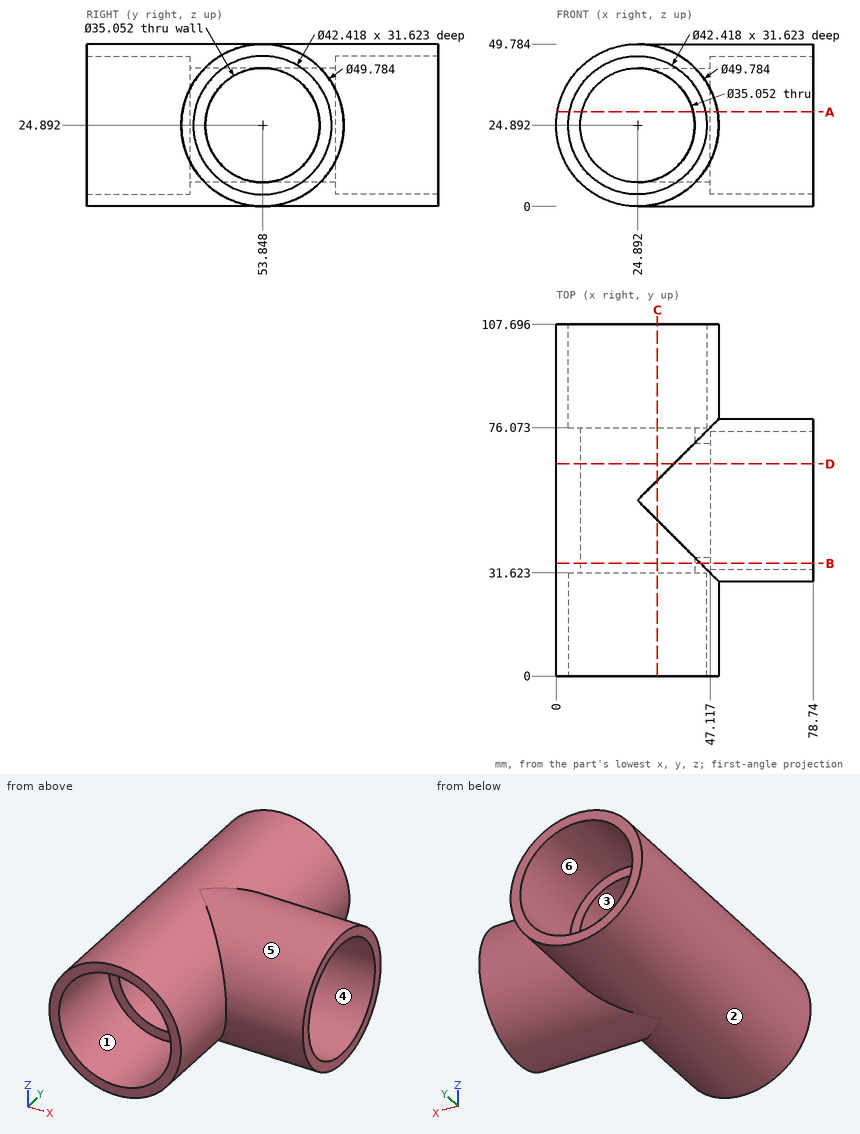
Drawing for the job (mm, zero at the part's lowest x, y, z). A direction names the side the tool comes from. Give positions to 0.01 mm unless a question says otherwise; leave off trailing zeros. Loops run counter-clockwise (first coordinate to the right, second up) from the corner with the lowest first, then second, coordinate; pieces in that order, holes last.
(1) Band-saw the part on A-A (z = 29). Write the cut outline in (x, y).
Return value:
outline: (0.34, 0) - (4.08, 0) - (4.08, 31.62) - (7.85, 31.62) - (7.85, 76.07) - (4.08, 76.07) - (4.08, 107.7) - (0.34, 107.7) - close; (41.93, 31.62) - (45.7, 31.62) - (45.7, 0) - (49.44, 0) - (49.44, 29.3) - (78.74, 29.3) - (78.74, 33.04) - (47.12, 33.04) - (47.12, 36.81) - (41.93, 36.81) - close; (41.93, 70.89) - (47.12, 70.89) - (47.12, 74.66) - (78.74, 74.66) - (78.74, 78.4) - (49.44, 78.4) - (49.44, 107.7) - (45.7, 107.7) - (45.7, 76.07) - (41.93, 76.07) - close
(2) Band-saw the part on C-C (x = 31). Write the cut outline in (y, z), and give its area (3 significant figures).
Return value:
outline: (0, 0.76) - (47.74, 0.76) arc R24.89 ccw to (59.96, 0.76) - (107.7, 0.76) - (107.7, 4.58) - (76.07, 4.58) - (76.07, 8.46) - (59.96, 8.46) arc R17.53 cw to (47.74, 8.46) - (31.62, 8.46) - (31.62, 4.58) - (0, 4.58) - close; (0, 45.2) - (31.62, 45.2) - (31.62, 41.32) - (47.74, 41.32) arc R17.53 cw to (59.96, 41.32) - (76.07, 41.32) - (76.07, 45.2) - (107.7, 45.2) - (107.7, 49.02) - (59.96, 49.02) arc R24.89 ccw to (47.74, 49.02) - (0, 49.02) - close
area: 1,160 mm2
(3) Drill centre lines: line 1 along X through (y, z) = (20, 25.5); line 2 along X through (y, z) = (70, 12); line 3 along Y through (x, z) = (55.5, 35). Where is each one in solid material? Low to high.
Return value:
line 1: x = 0.01 to 3.69, 46.09 to 49.78
line 2: x = 3.6 to 13.02, 36.76 to 47.12
line 3: y = 31.1 to 35.2, 72.49 to 76.6
(4) Pull direction Y, two halves, no side cores. Call the marked faces 4, 5 and 6: pulls with the +Y half, pulls with the -Y half, needs draft (parallel to the pull), parting line crosses it, or undercut.
Return value:
face 4: undercut
face 5: parting line crosses it
face 6: needs draft
(5) 3-axis set-ups, long thin cutter, end or side, ignore diameter. For the marked faces 1, 2 and 3: which of +Z, -Z, +X, -X, +Y, -Y reach the whole face in a straight line?
Return value:
face 1: -Y
face 2: none
face 3: +Y, -Y
(6) Pin check, flat tips, straight feed: pin 1 (21 mm diameter, centred on x = 30, z = 21, fed in from -Y); pin 2 (3 mm diameter, centred on y = 63.5, z = 10.5, fed in from -X); pin 3 (2 mm diameter, centred on y = 30.5, z = 13.5, fed in from +X); pin 4 (4 mm diameter, centred on x = 61, z = 44, fed in from +Y). Stop position of each tip, or through.
Return value:
pin 1: passes through
pin 2: stops at x = 3.6
pin 3: stops at x = 47.51
pin 4: stops at y = 71.93
(7) Band-saw the part on D-D (y = 65). Write the cut outline in (x, z).
Return value:
outline: (36.04, 2.64) - (78.74, 2.64) - (78.74, 6.85) - (47.12, 6.85) - (47.12, 11.37) - (36.04, 11.37) arc R17.53 cw (long way) to (36.04, 38.41) - (47.12, 38.41) - (47.12, 42.93) - (78.74, 42.93) - (78.74, 47.15) - (36.04, 47.15) arc R24.89 ccw (long way) to start
(8) Band-saw the part on B-B (y = 34.5). Write the cut outline in (x, z), and give its area (3 significant figures).
Return value:
outline: (44.24, 9.23) - (78.74, 9.23) - (78.74, 16.2) - (47.12, 16.2) - (47.12, 33.58) - (78.74, 33.58) - (78.74, 40.55) - (44.24, 40.55) arc R24.89 ccw (long way) to start; hole circle Ø35.05 at (24.89, 24.89)
area: 1,390 mm2
